The listing builds one solid part. Answer for the finished solid, in the listing's coordinates (mm). Round coordinates to 2 decimals unless told otherwise and drop trailing zeros. Order: outer loops, then holes, each group sorted by start corner. A loop starts at its lowest first (then second) coordinate and runs counter-clockwise, first axis right, second up. Notation, with made-up numbers: M -4.5,60 L 37.5,60 A23 ccw 37.5,68 Z; hole C 53,5.25 d7. An arc over 180 degrees is marked long. Write item = value, one per line. Start each with the question number.
(1) Each of these flat-tipped pins is pushed along its axis until it touches: pin 1 (3 mm diameter, centred on x = 4.5, y = 17.5, fed in from -Z); pin 2 (4 mm diameter, centred on y = 7.5, z = -4, fed in from -X); pin 3 (6 mm diameter, centred on x = 7.5, y = 17, fed in from +Z). Where does it stop, or does it pass through?
(2) A cutting plane is placed at B-B, the plane y = 2.25. Determine the outline of the cut face in (x, z), and give its area (3 significant figures).
(3) A cutting plane is placed at A-A, the plane y = 16.25. Determine the outline of the cut face in (x, z), and give its area (3 significant figures).
(4) Straight lines are drawn through the part: probe 1 along X at (y, z) = (3, 0); probe 2 along Y at (x, z) = (-5.75, -11); probe 3 along Z at (x, y) = (-6.25, 10.5). For each, find the intervals that lie inside material, in ascending order. Write a range as from..to.
from build123d import *

# Parameters (mm, degrees)
SKETCH1_R           = 13.5
BOSS_EXTRUDE1_DEPTH = 25
CHAMFER1_SIZE       = 6
FILLET1_R           = 3
FILLET2_R           = 1


with BuildPart() as part:
    # Sketch1 → Boss-Extrude1 (new body)
    with BuildSketch(Plane(origin=(0, 0, 0), x_dir=(1, 0, 0), z_dir=(0, 1, 0))):
        with Locations(Location((0, 0, 0), (0, 0, 270))):
            Circle(SKETCH1_R)
    extrude(amount=BOSS_EXTRUDE1_DEPTH)

    # Chamfer1
    chamfer1_edges = [part.edges().sort_by_distance(p)[0] for p in [
        (0, 25, -13.5),
    ]]
    chamfer(chamfer1_edges, length=CHAMFER1_SIZE)

    # Fillet1
    fillet1_edges = [part.edges().sort_by_distance(p)[0] for p in [
        (0, 0, -13.5),
    ]]
    fillet(fillet1_edges, radius=FILLET1_R)

    # Fillet2
    fillet2_edges = [part.edges().sort_by_distance(p)[0] for p in [
        (0, 25, -7.5),
        (0, 19, -13.5),
    ]]
    fillet(fillet2_edges, radius=FILLET2_R)


solid = part.part
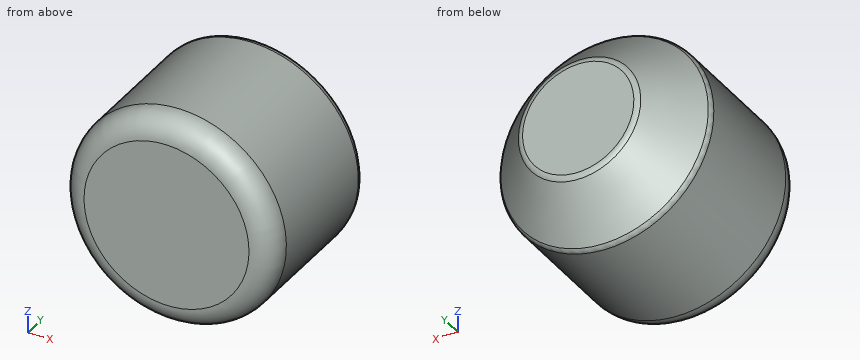
Reported:
q1.pin_1 = -13.16
q1.pin_2 = -13.35
q1.pin_3 = 12.73
q2.outline = C 0,0 d26.81
q2.area = 565 mm²
q3.outline = C 0,0 d27
q3.area = 573 mm²
q4.probe_1 = -13.5..13.5
q4.probe_2 = 0.69..20.09
q4.probe_3 = -11.97..11.97
